Build history of the part. All positions in model axes, mm. Give positions to 0.01 mm unless a question says otherwise; leave off trailing zeros. Write each loop counter-clockwise with the first axis right and the second up, starting at its lowest first coordinate (ties: lowest second). Pieces come first, ordered by that corner, then holes. Notation, with made-up numbers: M 51,88.25 L 71,88.25 A10 ccw 71,105.25 Z; hole C 51.5,58.5 d10. An arc over 180 degrees is marked long. Return JSON: item names as keys, results as strings. Group by question number.
Q1. Wall check: probe 1 along Z at (x, y) = (28, 1.25); probe 2 along Z at (x, y) = (22.5, 0.95); probe 3 along Z at (x, y) = (-1, 1.45). Give the ranges that are in metal, low to high.
Q2. Band-saw the part on D-D, the plane z = 43. Give the cut face in (x, y).
Q3. Band-saw the part on B-B, the plane z = 128.5. Give the cut face in (x, y), then the cut area to 3 significant figures.
Q4. Band-saw the part on A-A, the plane x = 1. Give the cut face in (y, z), then the cut area to 3 significant figures.
Q5. Band-saw the part on C-C, the plane y = 1.2. Count the separate pieces of the cut face and the enclosed holes in it, then the cut area to 3 significant figures.
Q6. Flat gauge pins, fed straight in: pin 1 Ø0.8 at (x, y) = (2, 1) entering from -Z; pin 2 Ø10 at (x, z) = (41.5, 146) entering from -Y; pin 3 Ø0.5 at (y, z) = (1, 137.5) entering from -X. Where does each tip first touch, or does it go through?
from build123d import *
from OCP.BRepFilletAPI import BRepFilletAPI_MakeFillet

# Parameters (mm, degrees)
SKETCH2_R           = 2.4
BOSS_EXTRUDE1_DEPTH = 1.57
FILLET1_R1          = 4
FILLET1_R2          = 6
FILLET2_R           = 2
SKETCH3_W           = 3
SKETCH3_H           = 6
SKETCH3_W_2         = 6
SKETCH3_H_2         = 3
CUT_EXTRUDE1_DEPTH  = 10


with BuildPart() as part:
    # Sketch2 → Boss-Extrude1 (new body)
    with BuildSketch(Plane(origin=(0, 0, 0), x_dir=(1, 0, 0), z_dir=(0, 1, 0))):
        with BuildLine():
            Line((-9.084283318, -126.509753408), (10.915716682, -126.509753408))
            Line((10.915716682, -126.509753408), (10.915716682, -160.509753408))
            Line((10.915716682, -160.509753408), (-9.084283318, -160.509753408))
            Line((-9.084283318, -160.509753408), (-9.084283318, -171.509753408))
            Line((-9.084283318, -171.509753408), (70.915716682, -171.509753408))
            Line((70.915716682, -171.509753408), (70.915716682, -160.509753408))
            Line((70.915716682, -160.509753408), (50.915716682, -160.509753408))
            Line((50.915716682, -160.509753408), (50.915716682, -126.509753408))
            Line((50.915716682, -126.509753408), (70.915716682, -126.509753408))
            Line((70.915716682, -126.509753408), (70.915716682, -48.669731747))
            Line((70.915716682, -48.669731747), (34.950716682, -48.669731747))
            Line((34.950716682, -48.669731747), (51.886612754, -20.102447618))
            ThreePointArc((51.886612754, -20.102447618), (51.921713055, -16.04745162), (48.415716682, -14.009753408))
            Line((48.415716682, -14.009753408), (13.415716682, -14.009753408))
            ThreePointArc((13.415716682, -14.009753408), (9.909720309, -16.04745162), (9.944820611, -20.102447618))
            Line((9.944820611, -20.102447618), (26.880716682, -48.669731747))
            Line((26.880716682, -48.669731747), (-9.084283318, -48.669731747))
            Line((-9.084283318, -48.669731747), (-9.084283318, -126.509753408))
        make_face()
        with Locations(Location((14.915716682, -167.509753408, 0), (0, 0, 270))):
            Circle(SKETCH2_R, mode=Mode.SUBTRACT)
        with Locations(Location((14.915716682, -151.509753408, 0), (0, 0, 270))):
            Circle(SKETCH2_R, mode=Mode.SUBTRACT)
        with Locations(Location((14.915716682, -135.509753408, 0), (0, 0, 270))):
            Circle(SKETCH2_R, mode=Mode.SUBTRACT)
        with Locations(Location((14.915716682, -119.509753408, 0), (0, 0, 270))):
            Circle(SKETCH2_R, mode=Mode.SUBTRACT)
        with BuildLine():
            ThreePointArc((18.915716682, -126.509753408), (19.794396339, -124.388433064), (21.915716682, -123.509753408))
            Line((21.915716682, -123.509753408), (39.915716682, -123.509753408))
            ThreePointArc((39.915716682, -123.509753408), (42.037037026, -124.388433064), (42.915716682, -126.509753408))
            Line((42.915716682, -126.509753408), (42.915716682, -160.509753408))
            ThreePointArc((42.915716682, -160.509753408), (42.037037026, -162.631073752), (39.915716682, -163.509753408))
            Line((39.915716682, -163.509753408), (21.915716682, -163.509753408))
            ThreePointArc((21.915716682, -163.509753408), (19.794396339, -162.631073752), (18.915716682, -160.509753408))
            Line((18.915716682, -160.509753408), (18.915716682, -126.509753408))
        make_face(mode=Mode.SUBTRACT)
        with Locations(Location((46.915716682, -167.509753408, 0), (0, 0, 270))):
            Circle(SKETCH2_R, mode=Mode.SUBTRACT)
        with Locations(Location((46.915716682, -147.509753408, 0), (0, 0, 270))):
            Circle(SKETCH2_R, mode=Mode.SUBTRACT)
        with Locations(Location((46.915716682, -135.509753408, 0), (0, 0, 270))):
            Circle(SKETCH2_R, mode=Mode.SUBTRACT)
        with Locations(Location((46.915716682, -119.509753408, 0), (0, 0, 270))):
            Circle(SKETCH2_R, mode=Mode.SUBTRACT)
        with Locations(Location((13.415716682, -18.044753408, 0), (0, 0, 270))):
            Circle(SKETCH2_R, mode=Mode.SUBTRACT)
        with Locations(Location((48.415716682, -18.044753408, 0), (0, 0, 270))):
            Circle(SKETCH2_R, mode=Mode.SUBTRACT)
    extrude(amount=BOSS_EXTRUDE1_DEPTH)

    # Fillet1: one fillet with a radius per group of edges: ONE call of the kernel's fillet builder (fillet() takes one radius for all edges)
    fillet1_edges_1 = [part.edges().sort_by_distance(p)[0] for p in [
        (50.915716682, 0.785, 126.509753408),
        (50.915716682, 0.785, 160.509753408),
        (10.915716682, 0.785, 126.509753408),
        (10.915716682, 0.785, 160.509753408),
    ]]
    fillet1_edges_2 = [part.edges().sort_by_distance(p)[0] for p in [
        (26.880716682, 0.785, 48.669731747),
        (34.950716682, 0.785, 48.669731747),
    ]]
    fillet1 = BRepFilletAPI_MakeFillet(part.part.solid().wrapped)
    for e in fillet1_edges_1:
        fillet1.Add(FILLET1_R1, e.wrapped)
    for e in fillet1_edges_2:
        fillet1.Add(FILLET1_R2, e.wrapped)
    add(Compound.cast(fillet1.Shape()), mode=Mode.REPLACE)

    # Fillet2
    fillet2_edges = [part.edges().sort_by_distance(p)[0] for p in [
        (70.915716682, 0.785, 48.669731747),
        (70.915716682, 0.785, 126.509753408),
        (70.915716682, 0.785, 160.509753408),
        (70.915716682, 0.785, 171.509753408),
        (-9.084283318, 0.785, 171.509753408),
        (-9.084283318, 0.785, 160.509753408),
        (-9.084283318, 0.785, 126.509753408),
        (-9.084283318, 0.785, 48.669731747),
    ]]
    fillet(fillet2_edges, radius=FILLET2_R)

    # Sketch3 → Cut-Extrude1 (cut)
    with BuildSketch(Plane(origin=(0, 1.57, 0), x_dir=(1, 0, 0), z_dir=(0, 1, 0))):
        with Locations((9.415716682, -166.009753408)):
            Rectangle(SKETCH3_W, SKETCH3_H)
        with Locations((52.415716682, -166.009753408)):
            Rectangle(SKETCH3_W, SKETCH3_H)
        with Locations((52.415716682, -121.009753408)):
            Rectangle(SKETCH3_W, SKETCH3_H)
        with Locations((9.415716682, -121.009753408)):
            Rectangle(SKETCH3_W, SKETCH3_H)
        with Locations((23.315716682, -67.009753408)):
            Rectangle(SKETCH3_W, SKETCH3_H)
        with Locations((38.515716682, -67.009753408)):
            Rectangle(SKETCH3_W, SKETCH3_H)
        with Locations((30.915716682, -82.509753408)):
            Rectangle(SKETCH3_W_2, SKETCH3_H_2)
    extrude(amount=-CUT_EXTRUDE1_DEPTH, mode=Mode.SUBTRACT)


solid = part.part
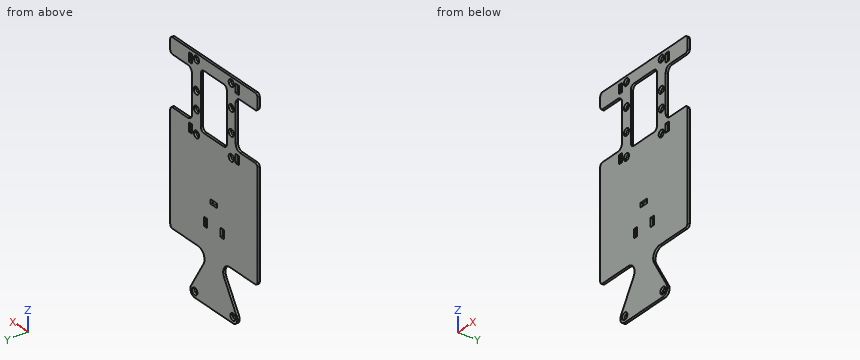
From the geometry:
{
 "1": {"probe 1": "z = 14.01 to 81.01, 84.01 to 123.51, 163.51 to 171.51", "probe 2": "z = 14.01 to 64.01, 70.01 to 123.51, 163.51 to 171.51", "probe 3": "z = 48.67 to 126.51, 160.51 to 171.51"},
 "2": {"outline": "M 22.34,0 L 39.49,0 L 39.49,1.57 L 22.34,1.57 Z"},
 "3": {"outline": "M 10.37,0 L 18.92,0 L 18.92,1.57 L 10.37,1.57 Z; M 42.92,0 L 51.46,0 L 51.46,1.57 L 42.92,1.57 Z", "area": "26.8 mm^2"},
 "4": {"outline": "M 0,48.67 L 1.57,48.67 L 1.57,126.51 L 0,126.51 Z; M 0,160.51 L 1.57,160.51 L 1.57,171.51 L 0,171.51 Z", "area": "139 mm^2"},
 "5": {"separate pieces": "1", "enclosed holes": "18", "area": "8,230 mm^2"},
 "6": {"pin 1": "stops at z = 48.67", "pin 2": "stops at y = 0", "pin 3": "stops at x = 10.92"}
}
